Source: CAD feature listing. Evaluate the final solid. Frame: model axes, mm. Give positions to 0.01 mm unless a question says otherwise; leave off trailing zeros. Write each loop counter-clockwise with the first axis right and the second up, starting at its lowest first coordinate (ties: lowest second). Pieces come first, ordered by that corner, then holes. Notation, with made-up numbers: (52, -25) -> (69, -25) arc R29 cw to (69, 6) -> close; hole circle Ø5 at (14, 6.25). An arc over 180 degrees is marked (long way). Use a Markdown table: item, result. Add a question column.
```python
from build123d import *

# Parameters (mm, degrees)
BOSS_EXTRUDE1_DEPTH = 4.3


with BuildPart() as part:
    # Sketch1 → Boss-Extrude1 (new body)
    with BuildSketch(Plane.XY):
        with BuildLine():
            Line((-335.7, -25), (-275.1, -25))
            Line((-275.1, -25), (-275.1, -29.3))
            Line((-275.1, -29.3), (-204.9, -29.3))
            Line((-204.9, -29.3), (-204.9, -25))
            Line((-204.9, -25), (-35.1, -25))
            Line((-35.1, -25), (-35.1, -29.3))
            Line((-35.1, -29.3), (35.1, -29.3))
            Line((35.1, -29.3), (35.1, -25))
            Line((35.1, -25), (48, -25))
            ThreePointArc((48, -25), (57.372583002, -2.372583002), (80, 7))
            Line((80, 7), (160, 7))
            ThreePointArc((160, 7), (182.627416998, -2.372583002), (192, -25))
            Line((192, -25), (204.9, -25))
            Line((204.9, -25), (204.9, -29.3))
            Line((204.9, -29.3), (275.1, -29.3))
            Line((275.1, -29.3), (275.1, -25))
            Line((275.1, -25), (335.7, -25))
            Line((335.7, -25), (335.7, -7.6))
            Line((335.7, -7.6), (340, -7.6))
            Line((340, -7.6), (340, 7.6))
            Line((340, 7.6), (335.7, 7.6))
            Line((335.7, 7.6), (335.7, 25))
            Line((335.7, 25), (275.1, 25))
            Line((275.1, 25), (275.1, 29.3))
            Line((275.1, 29.3), (204.9, 29.3))
            Line((204.9, 29.3), (204.9, 25))
            Line((204.9, 25), (35.1, 25))
            Line((35.1, 25), (35.1, 29.3))
            Line((35.1, 29.3), (-35.1, 29.3))
            Line((-35.1, 29.3), (-35.1, 25))
            Line((-35.1, 25), (-48, 25))
            ThreePointArc((-48, 25), (-57.372583002, 2.372583002), (-80, -7))
            Line((-80, -7), (-160, -7))
            ThreePointArc((-160, -7), (-182.627416998, 2.372583002), (-192, 25))
            Line((-192, 25), (-204.9, 25))
            Line((-204.9, 25), (-204.9, 29.3))
            Line((-204.9, 29.3), (-275.1, 29.3))
            Line((-275.1, 29.3), (-275.1, 25))
            Line((-275.1, 25), (-335.7, 25))
            Line((-335.7, 25), (-335.7, 7.6))
            Line((-335.7, 7.6), (-340, 7.6))
            Line((-340, 7.6), (-340, -7.6))
            Line((-340, -7.6), (-335.7, -7.6))
            Line((-335.7, -7.6), (-335.7, -25))
        make_face()
    extrude(amount=BOSS_EXTRUDE1_DEPTH)


solid = part.part
```
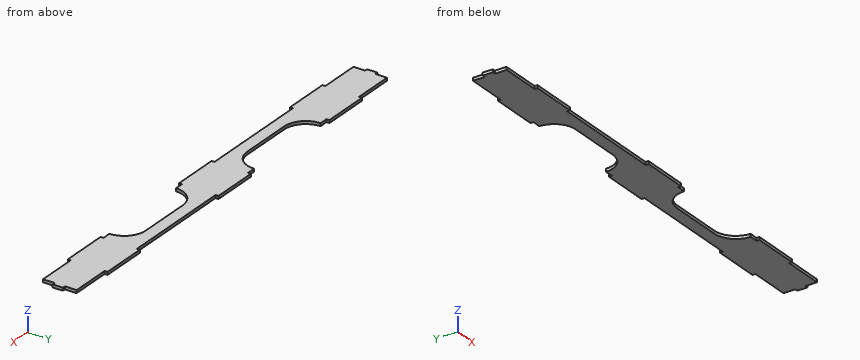
(1) Cut plane A-A on y = 17. Return the cut outline in (x, z).
(2) Cut plane B-B on x = 148. Return the cut outline in (y, z).
(3) First-contact query: pin 1 Ø1.5 at (y, z) = (-12.5, 2.5) entering from -X; pin 2 Ø2 at (x, z) = (299.5, 1.5) entering from -Y; pin 3 Ø2 at (y, z) = (-27, 2) entering from +X. Flat tips, straight axial feed; report the tip coordinate or a pass-through.
(4) Material intervals for L1, parallel to X at y = -26, z = 2.55; L2, parallel to X at y = -0.5, z = 2.75; L3, parallel to X at y = -22.5, z = 1.2, sorted ascending.
Output:
| question | item | result |
|---|---|---|
| 1 | outline | (-335.7, 0) -> (-190.98, 0) -> (-190.98, 4.3) -> (-335.7, 4.3) -> close; (-49.02, 0) -> (335.7, 0) -> (335.7, 4.3) -> (-49.02, 4.3) -> close |
| 2 | outline | (7, 0) -> (25, 0) -> (25, 4.3) -> (7, 4.3) -> close |
| 3 | pin 1 | x = -335.7 |
| 3 | pin 2 | y = -25 |
| 3 | pin 3 | x = 275.1 |
| 4 | L1 | -275.1 to -204.9, -35.1 to 35.1, 204.9 to 275.1 |
| 4 | L2 | -340 to -179.33, -60.67 to 59.41, 180.59 to 340 |
| 4 | L3 | -335.7 to 48.1, 191.9 to 335.7 |
